Check sheet for the modelled part. Datum: model origin and axes. Units: mm. A direction names the side the tool comes from. Give positions to 0.01 mm unless a question says otherwise; leave off trailing zeros. Order: outer loops, then holes, each group sorted by start corner. A loop starts at its lowest first (then second) coordinate and runs counter-clockwise, first axis right, second up. Notation, with made-up numbers: M -6.75,-10.75 L 38.25,-10.75 A30 cw 38.25,20.25 Z; hole C 60.5,72.25 d9. An arc over 180 degrees is marked long. Return JSON: item names as keys, results as strings. Group by question number.
from build123d import *

# Parameters (mm, degrees)
F0_R     = 3.5
F0_R_2   = 2.45
F1_DEPTH = 7.5
F2_R     = 5
F3_DEPTH = 5
F4_R     = 2.45
F5_DEPTH = 2.5


with BuildPart() as f1:
    # F0 (on Top) → F1 (new body)
    with BuildSketch(Plane.XY):
        Circle(F0_R)
        Circle(F0_R_2, mode=Mode.SUBTRACT)
    extrude(amount=F1_DEPTH)

    # F2 (on face) → F3 (join)
    with BuildSketch(Plane.XY.offset(7.5)):
        Circle(F2_R)
    extrude(amount=F3_DEPTH)

    # F4 (on face) → F5 (cut)
    with BuildSketch(Plane(origin=(0, 0, 7.5), x_dir=(1, 0, 0), z_dir=(0, 0, -1))):
        Circle(F4_R)
    extrude(amount=-F5_DEPTH, mode=Mode.SUBTRACT)


solid = f1.part
1) Sectioned sample at D-D on y = -3. Record the boundary of the cut face in (x, z), then the cut area to 3 significant figures.
2) Sectioned sample at C-C on z = 2. Record the boundary of the cut face in (x, y).
3) Tool access check on faces 5 (the face through (0, 0, 12.5)), 6 (the face through (3.233, -1.341, 3.698)). Record the directions out of +Z, -Z, +X, -X, +Y, -Y that give a thin tool (end or side, any length) a straight path to the whole face; none if there is none.
4) Sectioned sample at A-A on y = 0. Record the boundary of the cut face in (x, z), then the cut area to 3 significant figures.
5) Release check for a two-part mould opening along X. For faces 1 (the face through (0, 0, 10)), 2 (the face through (2.2, -3.3, 7.5)), 3 (the face through (-1.08, -4.88, 9.96)), 4 (the face through (-0.5, -2.4, 4.9)) record: released by +X, released by -X, zero draft, split by the parting line, or undercut.
6) Depth check by flat-ended pin: P1, Ø6, axis at x = -2, z = 3.5, coming from the +Y side. Enter the tip coordinate at first touch or a pass-through.
7) Material ranges on line 1 along Y through (x, z) = (0, 4.75); line 2 along Z through (x, y) = (3.25, -1.75); line 3 along Z through (x, y) = (-1.25, -1.25), recorded low to high.
Reply:
{
 "1": {"outline": "M -4,7.5 L -1.8,7.5 L -1.8,0 L 1.8,0 L 1.8,7.5 L 4,7.5 L 4,12.5 L -4,12.5 Z", "area": "67.0 mm^2"},
 "2": {"outline": "C 0,0 d7; hole C 0,0 d4.9"},
 "3": {"face 5": "+Z, +X, -X, +Y, -Y", "face 6": "-Z"},
 "4": {"outline": "M -5,7.5 L -3.5,7.5 L -3.5,0 L -2.45,0 L -2.45,10 L 2.45,10 L 2.45,0 L 3.5,0 L 3.5,7.5 L 5,7.5 L 5,12.5 L -5,12.5 Z", "area": "53.5 mm^2"},
 "5": {"face 1": "undercut", "face 2": "zero draft", "face 3": "split by the parting line", "face 4": "undercut"},
 "6": {"P1": "y = 3.5"},
 "7": {"line 1": "-3.5 to -2.45, 2.45 to 3.5", "line 2": "7.5 to 12.5", "line 3": "10 to 12.5"}
}
